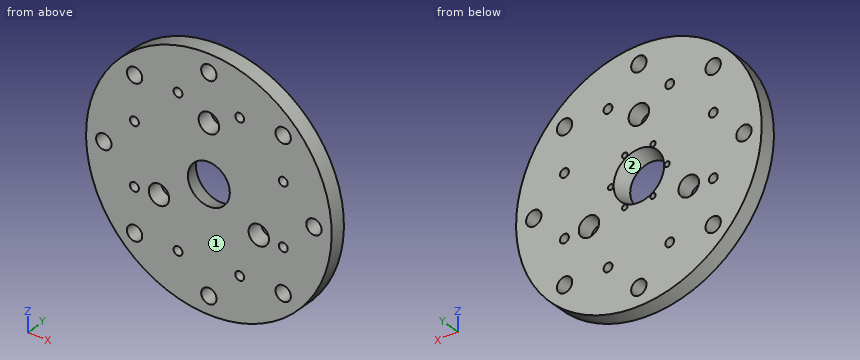
from build123d import *

# Parameters (mm, degrees)
SKETCH1_R                    = 76.2
BOSS_EXTRUDE1_DEPTH          = 10
SKETCH6_R                    = 2.75
CUT_EXTRUDE3_DEPTH           = 109.226059708
CIRPATTERN1_COUNT            = 8
SKETCH7_R                    = 6.35
CUT_EXTRUDE4_DEPTH           = 109.226059708
CIRPATTERN2_COUNT            = 3
F_3_8_0_375_DIAMETER_HOLE1_D = 9.525
CIRPATTERN4_COUNT            = 8
CIRPATTERN5_COUNT            = 6


with BuildPart() as part:
    # Sketch1 → Boss-Extrude1 (new body)
    with BuildSketch(Plane(origin=(0, 0, 0), x_dir=(1, 0, 0), z_dir=(0, 1, 0))):
        with Locations(Location((0, 0, 0), (0, 0, 270))):
            Circle(SKETCH1_R)
    extrude(amount=BOSS_EXTRUDE1_DEPTH)

    # Sketch5 → Cut-Revolve1 (revolve, cut)
    with BuildSketch(Plane.XY, mode=Mode.PRIVATE) as cut_revolve1_sk:
        Polygon((0, 0), (0, 10), (15.679491924, 10), (13, 0), align=None)
    revolve(cut_revolve1_sk.sketch.rotate(Axis((0, 0, 0), (0, 1, 0)), 90), axis=Axis((0, 0, 0), (0, 1, 0)), mode=Mode.SUBTRACT)

    # Sketch6 → Cut-Extrude3 (cut, through all)
    with BuildSketch(Plane(origin=(0, 0, 0), x_dir=(1, 0, 0), z_dir=(0, 1, 0))):
        with Locations(Location((46.193976626, 19.134171618, 0), (0, 0, 270))):
            Circle(SKETCH6_R)
    cut_extrude3 = extrude(amount=CUT_EXTRUDE3_DEPTH, mode=Mode.SUBTRACT)

    # CirPattern1: Cut-Extrude3 ×8 about axis
    cirpattern1_axis = Axis((0, 0, 0), (0, 1, 0))
    for i in range(1, CIRPATTERN1_COUNT):
        add(cut_extrude3.rotate(cirpattern1_axis, i * 360 / CIRPATTERN1_COUNT), mode=Mode.SUBTRACT)

    # Sketch7 → Cut-Extrude4 (cut, through all)
    with BuildSketch(Plane(origin=(0, 10, 0), x_dir=(1, 0, 0), z_dir=(0, 1, 0))):
        with Locations(Location((30.960408185, 17.875, 0), (0, 0, 270))):
            Circle(SKETCH7_R)
    cut_extrude4 = extrude(amount=-CUT_EXTRUDE4_DEPTH, mode=Mode.SUBTRACT)

    # CirPattern2: Cut-Extrude4 ×3 about axis
    cirpattern2_axis = Axis((0, 0, 0), (0, 1, 0))
    for i in range(1, CIRPATTERN2_COUNT):
        add(cut_extrude4.rotate(cirpattern2_axis, i * 360 / CIRPATTERN2_COUNT), mode=Mode.SUBTRACT)

    # 3/8 (0.375) Diameter Hole1 (through all)
    with Locations(Plane(origin=(0, 10, 0), x_dir=(1, 0, 0), z_dir=(0, 1, 0))):
        with Locations((-65.2, 0)):
            f_3_8_0_375_diameter_hole1 = Hole(F_3_8_0_375_DIAMETER_HOLE1_D / 2)

    # CirPattern4: 3/8 (0.375) Diameter Hole1 ×8 about axis
    cirpattern4_axis = Axis((0, 0, 0), (0, 1, 0))
    for i in range(1, CIRPATTERN4_COUNT):
        add(f_3_8_0_375_diameter_hole1.rotate(cirpattern4_axis, i * 360 / CIRPATTERN4_COUNT), mode=Mode.SUBTRACT)

    # Sketch13 → Tap Drill for M4x0.7 Tap1 (revolve, cut)
    with BuildSketch(Plane(origin=(17.5, 10, 0), x_dir=(0, 0, 1), z_dir=(1, 0, 0))):
        Polygon((0, 0), (0, 8.991420021), (1.65, 8), (1.65, 0), align=None)
    tap_drill_for_m4x0_7_tap1 = revolve(axis=Axis((17.5, 16.35, 0), (0, -1, 0)), mode=Mode.SUBTRACT)

    # CirPattern5: Tap Drill for M4x0.7 Tap1 ×6 about axis
    cirpattern5_axis = Axis((0, 0, 0), (0, 1, 0))
    for i in range(1, CIRPATTERN5_COUNT):
        add(tap_drill_for_m4x0_7_tap1.rotate(cirpattern5_axis, i * 360 / CIRPATTERN5_COUNT), mode=Mode.SUBTRACT)


solid = part.part
Source: CAD feature listing. Evaluate the final solid. Frame: model axes, mm. Face numbers are marked on the shaded views. Give positions to 0.01 mm unless a question says otherwise; leave off trailing zeros. Write each loop counter-clockwise with the first axis right and the second up, starting at its lowest first coordinate (ties: lowest second). Pieces come first, ordered by that corner, then holes. Notation, with made-up numbers: (32.5, -2.5) -> (84.5, -2.5) arc R33 cw to (84.5, 29.5) -> close; hole circle Ø3 at (-39.75, -2.5). An arc over 180 degrees is marked (long way). Write item = value, one per line.
Q1. Cut plane C-C on y = 5. State how many separate pieces and enclosed holes the cut face has, then the cut area to 3 significant figures.
Here are the results:
separate_pieces = 1
enclosed_holes = 26
area = 16,400 mm²
Q2. Cut plane A-A on x = 0. Return loops of the section in (y, z), then the cut area to 3 significant figures.
Here are the results:
outline = (0, -76.2) -> (10, -76.2) -> (10, -69.96) -> (0, -69.96) -> close; (0, -60.44) -> (10, -60.44) -> (10, -15.68) -> (0, -13) -> close; (0, 13) -> (10, 15.68) -> (10, 29.4) -> (0, 29.4) -> close; (0, 42.1) -> (10, 42.1) -> (10, 60.44) -> (0, 60.44) -> close; (0, 69.96) -> (10, 69.96) -> (10, 76.2) -> (0, 76.2) -> close
area = 920 mm²
Q3. Mould query, pull axis X, two halves, no side actions, for the marked faces 1 and 2. Classes: +X half, -X half, draft (parallel to the pull), parting line (faces both ways), or undercut.
Here are the results:
face_1 = draft
face_2 = undercut
Q4. Cut plane B-B on z = -65. Return loops of the section in (x, y).
Here are the results:
outline = (-39.77, 0) -> (-4.76, 0) -> (-4.76, 10) -> (-39.77, 10) -> close; (4.76, 0) -> (39.77, 0) -> (39.77, 10) -> (4.76, 10) -> close
Q5. Cut plane D-D on z = 65.2. Return loops of the section in (x, y).
Here are the results:
outline = (-39.44, 0) -> (-4.76, 0) -> (-4.76, 10) -> (-39.44, 10) -> close; (4.76, 0) -> (39.44, 0) -> (39.44, 10) -> (4.76, 10) -> close
Q6. First-contact query: pin 1 (6 mm diameter, centred on y = 4, z = 6, fed in from +X); pin 2 (5.5 mm diameter, centred on x = 46.1, z = 46.1, fed in from -Y); pin 3 (3 mm diameter, centred on x = -32, y = 8.5, fed in from -Z); pin 4 (1 mm diameter, centred on y = 3.5, z = -16, fed in from -X). Flat tips, straight axial feed; report the tip coordinate or a pass-through.
Here are the results:
pin_1 = 76.14
pin_2 = through
pin_3 = -69.83
pin_4 = -74.61
Q7. Line query: line 1 (X direction, y = 3.75, z = 47); line 2 (Z direction, x = 7.5, y = 2.75); line 3 (Z direction, x = 48.5, y = 2). Output: solid intervals per line, ascending. Write a range as from..to.
Here are the results:
line_1 = -59.98..-50.78, -41.43..-21.76, -16.5..16.5, 21.76..41.43, 50.78..59.98
line_2 = -75.83..-16.23, -14.08..-11.51, 11.51..14.08, 16.23..75.83
line_3 = -58.77..-50.22, -41.99..-20.63, -17.64..17.64, 20.63..41.99, 50.22..58.77
